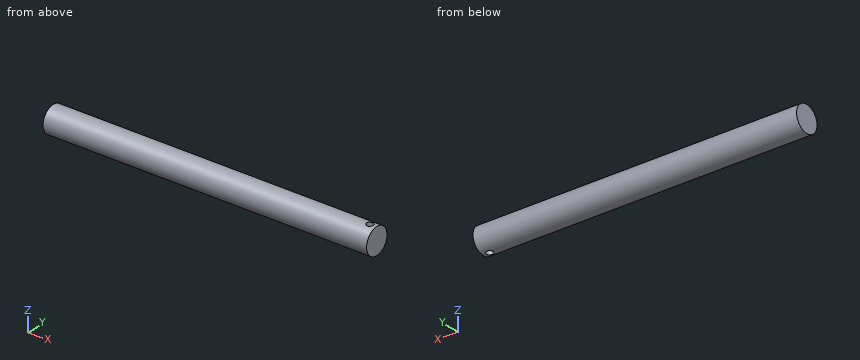
from build123d import *

# Parameters (mm, degrees)
SKETCH1_R               = 4.85
BOSS_EXTRUDE1_DEPTH     = 120
CUT_EXTRUDE1_DEPTH      = 121.195860994
CUT_EXTRUDE1_DEPTH_BACK = 121.195860994
SKETCH2_R               = 1.25
SCALE1_SCALE            = 1.5


with BuildPart() as part:
    # Sketch1 → Boss-Extrude1 (new body)
    with BuildSketch(Plane(origin=(0, 0, 0), x_dir=(0, 0, -1), z_dir=(1, 0, 0))):
        Circle(SKETCH1_R)
    extrude(amount=BOSS_EXTRUDE1_DEPTH)

    # Sketch2 → Cut-Extrude1 (cut, two sides: drawn at the far end of the back side and taken through both)
    with BuildSketch(Plane.XY.offset(-CUT_EXTRUDE1_DEPTH_BACK)):
        with Locations((117.5, 0)):
            Circle(SKETCH2_R)
    extrude(amount=CUT_EXTRUDE1_DEPTH + CUT_EXTRUDE1_DEPTH_BACK, mode=Mode.SUBTRACT)


with BuildPart() as part_1:
    # Scale1: scaled about (59.692221028, 5e-09, 2.22e-07)
    add(part.part.scale(SCALE1_SCALE).moved(Location((-29.846110514, -3e-09, -1.11e-07))))


solid = part_1.part
Check sheet for the modelled part. Datum: model origin and axes. Units: mm. Give positions to 0.01 mm unless a question says otherwise; leave off trailing zeros. Loops run counter-clockwise (first coordinate to the right, second up) from the corner with the lowest first, then second, coordinate; pieces in that order, holes last. Notation, with made-up numbers: M 6,10.5 L 25,10.5 A25 cw 25,31.5 Z; hole C -31,-15 d8. An arc over 180 degrees is marked long. Use a Markdown table: item, result. Add a question column.
Q1. Sectioned sample at B-B, the plane z = -5.75. Record the cut outline in (x, y) (3 decimals), then the cut area to 3 significant figures.
Q2. Go/stop test with flat-tipped pins: pin 1 (3.5 mm diameter, centred on x = 146.4, y = 0, fed in from -Z); pin 2 (6 mm diameter, centred on x = 30, y = 4.5, fed in from -Z); pin 3 (1 mm diameter, centred on x = 21, z = -3.5, fed in from -Y). Record where each tip stops, or that it passes through.
Q3. Scan lines: line 1 along X through (y, z) = (-0.25, 0.25); line 2 along X through (y, z) = (-1, -3); line 3 along Y through (x, z) = (91, -0.5). Record each from-to range of solid material in increasing order. Write a range as [from, to].
Q4. Sectioned sample at C-C, the plane z = 4.5. Record the cut outline in (x, y) (3 decimals).
Q5. Sectioned sample at A-A, the plane y = 0. Record the cut outline in (x, z) (3 decimals).
Verdict:
| question | item | result |
|---|---|---|
| 1 | outline | M -29.846,-4.457 L 150.154,-4.457 L 150.154,4.457 L -29.846,4.457 Z; hole C 146.404,0 d3.75 |
| 1 | area | 1,590 mm^2 |
| 2 | pin 1 | through |
| 2 | pin 2 | z = -7.12 |
| 2 | pin 3 | y = -6.63 |
| 3 | line 1 | [-29.85, 144.55], [148.26, 150.15] |
| 3 | line 2 | [-29.85, 144.82], [147.99, 150.15] |
| 3 | line 3 | [-7.26, 7.26] |
| 4 | outline | M -29.846,-5.716 L 150.154,-5.716 L 150.154,5.716 L -29.846,5.716 Z; hole C 146.404,0 d3.75 |
| 5 | outline | M -29.846,-7.275 L 144.529,-7.275 L 144.529,7.275 L -29.846,7.275 Z; M 148.279,-7.275 L 150.154,-7.275 L 150.154,7.275 L 148.279,7.275 Z |
